from build123d import *

# Parameters (mm, degrees)
BOSS_EXTRUDE1_DEPTH = 75
SKETCH8_R           = 95
SKETCH8_R_2         = 70
CUT_EXTRUDE6_DEPTH  = 10
SKETCH9_R           = 5
CUT_EXTRUDE7_DEPTH  = 10
BOSS_EXTRUDE2_DEPTH = 75
CUT_EXTRUDE10_DEPTH = 108.26147997


with BuildPart() as part:
    # Sketch1 → Boss-Extrude1 (new body)
    with BuildSketch(Plane(origin=(0, 0, 0), x_dir=(1, 0, 0), z_dir=(0, 1, 0))):
        with BuildLine():
            Line((-58, 0), (57, 0))
            Line((57, 0), (57, 8.158918194))
            ThreePointArc((57, 8.158918194), (56.905987413, 8.764898378), (56.632788017, 9.313908796))
            Line((56.632788017, 9.313908796), (42.597737063, 29.154990602))
            ThreePointArc((42.597737063, 29.154990602), (41.884192973, 29.776229321), (40.964949045, 30))
            Line((40.964949045, 30), (2, 30))
            ThreePointArc((2, 30), (0.585786438, 29.414213562), (0, 28))
            Line((0, 28), (0, 27))
            ThreePointArc((0, 27), (-0.585786438, 25.585786438), (-2, 25))
            Line((-2, 25), (-41, 25))
            ThreePointArc((-41, 25), (-42.414213562, 25.585786438), (-43, 27))
            Line((-43, 27), (-43, 33))
            ThreePointArc((-43, 33), (-43.585786438, 34.414213562), (-45, 35))
            Line((-45, 35), (-58, 35))
            Line((-58, 35), (-58, 0))
        make_face()
    extrude(amount=BOSS_EXTRUDE1_DEPTH)

    # Sketch8 → Cut-Extrude6 (cut)
    with BuildSketch(Plane(origin=(0, 75, 0), x_dir=(1, 0, 0), z_dir=(0, 1, 0))):
        with Locations((57, 0)):
            Circle(SKETCH8_R)
        with Locations((57, 0)):
            Circle(SKETCH8_R_2, mode=Mode.SUBTRACT)
    extrude(amount=-CUT_EXTRUDE6_DEPTH, mode=Mode.SUBTRACT)

    # Sketch9 → Cut-Extrude7 (cut)
    with BuildSketch(Plane(origin=(0, 65, 0), x_dir=(1, 0, 0), z_dir=(0, 1, 0))):
        with Locations((-26, 0)):
            Circle(SKETCH9_R)
        with Locations(Location((-24.633326528, 15, 0), (0, 0, 270))):
            Circle(SKETCH9_R)
    extrude(amount=-CUT_EXTRUDE7_DEPTH, mode=Mode.SUBTRACT)

    # Sketch11 → Boss-Extrude2 (add)
    with BuildSketch(Plane(origin=(0, 75, 0), x_dir=(1, 0, 0), z_dir=(0, 1, 0))):
        with BuildLine():
            Line((-68.227744249, 0), (-58, 0))
            Line((-58, 0), (-58, 35))
            ThreePointArc((-58, 35), (-65.618435157, 18.231886576), (-68.227744249, 0))
        make_face()
    extrude(amount=-BOSS_EXTRUDE2_DEPTH)

    # Sketch12 → Cut-Extrude10 (cut, through all)
    with BuildSketch(Plane.XY):
        Polygon((57, 0), (-68.227744249, 0), (-18, 45), (57, 45), align=None)
    extrude(amount=-CUT_EXTRUDE10_DEPTH, mode=Mode.SUBTRACT)


solid = part.part
The model under review builds one solid part; all positions refer to its coordinate system, in mm. A direction names the side the tool comes from. Round coordinates to 2 decimals unless told otherwise and drop trailing zeros. Loops run counter-clockwise (first coordinate to the right, second up) from the corner with the lowest first, then second, coordinate; pieces in that order, holes last. Notation, with made-up numbers: M -25.5,66 L 6.5,66 A8 cw 6.5,72 Z; hole C 41.25,19 d7. An arc over 180 degrees is marked long. Answer as a JSON object with one key per item and string values.
Item 1: We need section D-D, the plane y = 6. State the section outline as (x, z) points.
Check sheet entries:
{"outline": "M -68.23,0 A65 ccw -61.53,-28.74 L -61.53,0 Z"}
Item 2: Clearance check with flat-ended pins moving along their axes: P1, Ø2.5, axis at x = -23.5, z = -2, coming from the +Y side; P2, Ø9, axis at x = 21.5, y = 63, coming from the -Z side; P3, Ø5, axis at x = -31.5, z = -12.5, coming from the -Y side. State where each tip first meets the part, or that it passes through.
Check sheet entries:
{"P1": "y = 55", "P2": "z = -30", "P3": "y = 30.67"}
Item 3: We need section A-A, the plane x = 12. State the section outline as (y, z) points, and give its area (3 significant figures).
Check sheet entries:
{"outline": "M 45,-30 L 75,-30 L 75,0 L 45,0 Z", "area": "900 mm2"}
Item 4: Tool access review of faces 4 (the face through (-37.135, 70.07, -12.787)), 5 (the face through (-29.514, 60.07, -16.084)), 6 (the face through (-43, 48, -30)), 7 (the face through (19, 45, -15)): name each direction out of +Z, -Z, +X, -X, +Y, -Y from which nothing blocks a thin tool from reaching the whole face with its end or side.
Check sheet entries:
{"face 4": "+Z, +Y", "face 5": "+Y", "face 6": "-Z, +Y, -Y", "face 7": "+Z, -Z, +X, -Y"}
Item 5: The part is to be moulded in two halves that separate along X. For faces 1 (the face through (57, 60, -4)), 2 (the face through (-26, 55, -2)), 3 (the face through (-51, 42, -35)), say which applies: +X half, -X half, draft (parallel to the pull), parting line (faces both ways), or undercut.
Check sheet entries:
{"face 1": "+X half", "face 2": "undercut", "face 3": "draft"}
Item 6: We need section B-B, the plane y = 60. State the section outline as (x, z) points (3 decimals).
Check sheet entries:
{"outline": "M -68.228,0 A65 ccw -58,-35 L -45,-35 A2 ccw -43,-33 L -43,-27 A2 cw -41,-25 L -2,-25 A2 cw 0,-27 L 0,-28 A2 ccw 2,-30 L 40.965,-30 A2 ccw 42.598,-29.155 L 56.633,-9.314 A2 ccw 57,-8.159 L 57,0 L -21,0 A5 cw -31,0 Z; hole C -24.633,-15 d10"}
Item 7: We need section C-C, the plane z = -15. State the section outline as (x, y) points, and give its area (3 significant figures).
Check sheet entries:
{"outline": "M -66.47,1.57 L -18,45 L 52.61,45 L 52.61,75 L -11.37,75 L -11.37,65 L -19.63,65 L -19.63,55 L -29.63,55 L -29.63,65 L -36.81,65 L -36.81,75 L -66.47,75 Z", "area": "4,270 mm2"}
Item 8: For line 1 along Y through (x, z) = (0.5, -8.5); line 2 along Z through (x, y) = (-36, 43); line 3 along X through (y, z) = (58, -19), list the stretches that pass through material, from the lowest coordinate up.
Check sheet entries:
{"line 1": "45 to 75", "line 2": "-25 to 0", "line 3": "-65.39 to -27.63, -21.63 to 49.78"}
